Here's how the part is built. I have some questions about the finished solid (model axes, mm). Give positions to 0.01 mm unless a question says otherwise; leave off trailing zeros. Loops run counter-clockwise (first coordinate to the right, second up) from the corner with the lowest first, then second, coordinate; pieces in that order, holes last.
Q1. If we section it at C-C (z = 2.8): Please give me the cut outline in (x, y).
Q2. Will this pin go through, and if not, where does the flat tip stop? P1, Ø1.5, axis at y = 1, z = 2, coming from the -X side.
Q3. If we section it at A-A (x = 0): Please give me the cut outline in (y, z).
Q4. We'd pull the mould along X, two halves only. Please class faces 1 (the face through (0.64, 2.88, 2.11)), 2 (the face through (2, -1, 0)), 3 (the face through (0.37, -1.66, 1.58)): +X half, -X half, draft (parallel to the pull), parting line (faces both ways), or undercut.
Q5. I need wall thicknesses on line 1 (Y direction, x = 0, z = 2.05); line 2 (Y direction, x = -1.25, z = 0.35); line 3 (X direction, y = -0.25, z = 0.45). Which ranges of each line are inside material? Lowest first, please.
from build123d import *

# Parameters (mm, degrees)
HOLE_WIZARD_M3_1_D           = 3.4
HOLE_WIZARD_M3_1_CBORE_D     = 9
HOLE_WIZARD_M3_1_CBORE_DEPTH = 0.5
FILLET_2_R                   = 0.3


with BuildPart() as part:
    # 草图1 → 旋转1 (revolve)
    with BuildSketch(Plane(origin=(0, 0, 0), x_dir=(0, 0, -1), z_dir=(1, 0, 0)), mode=Mode.PRIVATE) as revolve_1_sk:
        with BuildLine():
            Line((0, 0), (0, -3.509931985))
            ThreePointArc((0, -3.509931985), (-0.081099311, -3.643171225), (-0.236702601, -3.632335658))
            Line((-0.236702601, -3.632335658), (-1.122080957, -3.005192656))
            ThreePointArc((-1.122080957, -3.005192656), (-1.204497707, -2.964130971), (-1.295486159, -2.95))
            Line((-1.295486159, -2.95), (-3.4, -2.95))
            ThreePointArc((-3.4, -2.95), (-3.612132034, -2.862132034), (-3.7, -2.65))
            Line((-3.7, -2.65), (-3.7, 0))
            Line((-3.7, 0), (0, 0))
        make_face()
    revolve(revolve_1_sk.sketch.rotate(Axis((0, 0, 0), (0, 0, 1)), 270), axis=Axis((0, 0, 0), (0, 0, 1)))

    # M3 六角头螺栓的柱形沉头孔1 (through all)
    with Locations(Plane.XY.offset(3.7)):
        with Locations((0, 0)):
            CounterBoreHole(HOLE_WIZARD_M3_1_D / 2, HOLE_WIZARD_M3_1_CBORE_D / 2, HOLE_WIZARD_M3_1_CBORE_DEPTH)

    # 圆角2
    fillet_2_edges = [part.edges().sort_by_distance(p)[0] for p in [
        (2.95, 0, 3.2),
    ]]
    fillet(fillet_2_edges, radius=FILLET_2_R)


solid = part.part
Check sheet entries:
1. outline: circle Ø5.9 at (0, 0); hole circle Ø3.4 at (0, 0)
2. P1: stops at x = -2.94
3. outline: (-3.63, 0.24) arc R0.15 ccw to (-3.51, 0) - (-1.7, 0) - (-1.7, 3.2) - (-2.65, 3.2) arc R0.3 ccw to (-2.95, 2.9) - (-2.95, 1.3) arc R0.3 cw to (-3.01, 1.12) - close; (1.7, 0) - (3.51, 0) arc R0.15 ccw to (3.63, 0.24) - (3.01, 1.12) arc R0.3 cw to (2.95, 1.3) - (2.95, 2.9) arc R0.3 ccw to (2.65, 3.2) - (1.7, 3.2) - close
4. face 1: parting line
4. face 2: draft
4. face 3: undercut
5. line 1: y = -2.95 to -1.7, 1.7 to 2.95
5. line 2: y = -3.32 to -1.15, 1.15 to 3.32
5. line 3: x = -3.47 to -1.68, 1.68 to 3.47
